```python
from build123d import *

# Parameters (mm, degrees)
SKETCH_1_R          = 3.1
SKETCH_1_R_2        = 1.6
SKETCH_1_W          = 20.4
SKETCH_1_H          = 40.4
EXTRUDE_1_DEPTH     = 4
FILLET_1_R          = 0.2
SKETCH_2_R          = 2.1
CUT_EXTRUDE_1_DEPTH = 4
CUT_EXTRUDE_2_DEPTH = 10
SKETCH_4_W          = 44.796452611
SKETCH_4_H          = 12
CUT_EXTRUDE_3_DEPTH = 10
FILLET_2_R          = 6


with BuildPart() as part:
    # 草图1 → 凸台-拉伸1 (new body)
    with BuildSketch(Plane.XY):
        with BuildLine():
            Line((-13.2, 27), (60.15625, 27))
            ThreePointArc((60.15625, 27), (63.954895943, 25.251198086), (65.096310169, 21.228115599))
            Line((65.096310169, 21.228115599), (62.440060169, 4.228115599))
            ThreePointArc((62.440060169, 4.228115599), (61.816569536, 2.476663431), (60.596300169, 1.074070141))
            Line((60.596300169, 1.074070141), (27.72371786, -24.851859719))
            ThreePointArc((27.72371786, -24.851859719), (24.808418455, -26.447713935), (21.531117522, -27))
            Line((21.531117522, -27), (-13.2, -27))
            ThreePointArc((-13.2, -27), (-20.271067812, -24.071067812), (-23.2, -17))
            Line((-23.2, -17), (-23.2, 17))
            ThreePointArc((-23.2, 17), (-20.271067812, 24.071067812), (-13.2, 27))
        make_face()
        with Locations((33, 2)):
            Circle(SKETCH_1_R, mode=Mode.SUBTRACT)
        with Locations((60, 21)):
            Circle(SKETCH_1_R_2, mode=Mode.SUBTRACT)
        with Locations((57.5, 5)):
            Circle(SKETCH_1_R_2, mode=Mode.SUBTRACT)
        Rectangle(SKETCH_1_W, SKETCH_1_H, mode=Mode.SUBTRACT)
    extrude(amount=EXTRUDE_1_DEPTH)

    # 圆角1
    fillet_1_edges = [part.edges().sort_by_distance(p)[0] for p in [
        (-10.2, 20.2, 2),
        (-10.2, -20.2, 2),
        (10.2, -20.2, 2),
        (10.2, 20.2, 2),
    ]]
    fillet(fillet_1_edges, radius=FILLET_1_R)

    # 草图2 → 切除-拉伸1 (cut)
    with BuildSketch(Plane.XY.offset(4)):
        with Locations((14.95, 11)):
            Circle(SKETCH_2_R)
        with Locations(Location((14.95, -11, 0), (0, 0, 180))):
            Circle(SKETCH_2_R)
        with Locations((-17.95, -11)):
            Circle(SKETCH_2_R)
        with Locations(Location((-17.95, 11, 0), (0, 0, 180))):
            Circle(SKETCH_2_R)
    extrude(amount=-CUT_EXTRUDE_1_DEPTH, mode=Mode.SUBTRACT)

    # 草图3 → 切除-拉伸2 (cut)
    with BuildSketch(Plane.XY.offset(4)):
        with BuildLine():
            Line((25.798016292, 21), (51.43418263, 21))
            ThreePointArc((51.43418263, 21), (53.713370196, 19.950718852), (54.398218731, 17.536869359))
            Line((54.398218731, 17.536869359), (52.852232934, 7.642560256))
            ThreePointArc((52.852232934, 7.642560256), (51.264559821, 5.440053089), (48.549531682, 5.420923567))
            Line((48.549531682, 5.420923567), (24.905572858, 17.210155114))
            ThreePointArc((24.905572858, 17.210155114), (23.851263897, 19.458426781), (25.798016292, 21))
        make_face()
    extrude(amount=-CUT_EXTRUDE_2_DEPTH, mode=Mode.SUBTRACT)

    # 草图4 → 切除-拉伸3 (cut)
    with BuildSketch(Plane.XY.offset(4)):
        with Locations((43.929343828, -21)):
            Rectangle(SKETCH_4_W, SKETCH_4_H)
    extrude(amount=-CUT_EXTRUDE_3_DEPTH, mode=Mode.SUBTRACT)

    # 圆角2
    fillet_2_edges = [part.edges().sort_by_distance(p)[0] for p in [
        (40.215307217, -15, 2),
        (21.531117522, -27, 2),
        (21.531117522, -15, 2),
    ]]
    fillet(fillet_2_edges, radius=FILLET_2_R - 0.0001)  # a hair under: the kernel refuses the full size


solid = part.part
```
Check sheet for the modelled part. Datum: model origin and axes. Units: mm. A direction names the side the tool comes from. Give positions to 0.01 mm unless a question says otherwise; leave off trailing zeros. Write each loop counter-clockwise with the first axis right and the second up, starting at its lowest first coordinate (ties: lowest second). Pieces come first, ordered by that corner, then holes. Notation, with made-up numbers: (78.25, -18) -> (134.25, -18) arc R18 ccw to (134.25, 15) -> close; hole circle Ø11 at (61, -3). An arc over 180 degrees is marked (long way). Use CSV: the item, a comma, the result in double quotes. Start each with the question number.
Q1. Release check for a two-part mould opening along X. For faces 3 (the flat face through (22, 6, 4)), 4 (the cylindrical face through (23.843, 19.422, 2.028)), 5 (the cylindrical face through (63.915, 25.297, 1.972)), 6 (the flat face through (0, -20.2, 2)) record: +X half, -X half, draft (parallel to the pull), parting line (faces both ways), or undercut.
Q2. Scan lines: line 1 along Y through (x, z) = (14.95, 3); line 2 along Y through (x, z) = (-10, 2.45); line 3 along Y through (x, z) = (-17.95, 1.85). Record each from-to range of solid material in increasing order.
Q3. Cross-section at B-B on x = 57.5. Enter the section's corners in (y, z), and give its area (3 significant figures).
Q4. Tool access check on faces 1 (the flat face through (-23.2, 0, 2)), 2 (the cylindrical face through (53.69, 19.98, 2.03)). Record the directions out of +Z, -Z, +X, -X, +Y, -Y that give a thin tool (end or side, any length) a straight path to the whole face; none if there is none.
Q5. Cross-section at D-D on x = -17.95. Enter the section's corners in (y, z), and give its area (3 significant figures).
Q6. Depth check by flat-ended pin: P1, Ø2, axis at y = -6, z = 2.5, coming from the +X side; P2, Ø3.5, axis at x = 33, y = 2, coming from the -Z side; P3, Ø1, axis at y = -20.5, z = 0.5, coming from the -X side; P4, Ø2, axis at y = 11.5, z = 1, coming from the +X side. Enter the tip coordinate at first touch or a pass-through.
Q7. Cross-section at C-C on y = 11. Enter the section's corners in (x, z), and give its area (3 significant figures).
Q8. Cross-section at A-A on y = -11. Enter the section's corners in (x, z), and give its area (3 significant figures).
Working result:
1,face 3,"draft"
1,face 4,"undercut"
1,face 5,"+X half"
1,face 6,"undercut"
2,line 1,"y = -27 to -13.1, -8.9 to 8.9, 13.1 to 27"
2,line 2,"y = -27 to -20.2, 20.2 to 27"
2,line 3,"y = -25.8 to -13.1, -8.9 to 8.9, 13.1 to 25.8"
3,outline,"(-1.37, 0) -> (3.4, 0) -> (3.4, 4) -> (-1.37, 4) -> close; (6.6, 0) -> (27, 0) -> (27, 4) -> (6.6, 4) -> close"
3,area,"101 mm^2"
4,face 1,"+Z, -Z, -X, +Y, -Y"
4,face 2,"+Z, -Z"
5,outline,"(-25.8, 0) -> (-13.1, 0) -> (-13.1, 4) -> (-25.8, 4) -> close; (-8.9, 0) -> (8.9, 0) -> (8.9, 4) -> (-8.9, 4) -> close; (13.1, 0) -> (25.8, 0) -> (25.8, 4) -> (13.1, 4) -> close"
5,area,"173 mm^2"
6,P1,"stops at x = 52.89"
6,P2,"passes through"
6,P3,"stops at x = -22.74"
6,P4,"stops at x = 63.73"
7,outline,"(-23.2, 0) -> (-20.05, 0) -> (-20.05, 4) -> (-23.2, 4) -> close; (-15.85, 0) -> (-10.2, 0) -> (-10.2, 4) -> (-15.85, 4) -> close; (10.2, 0) -> (12.85, 0) -> (12.85, 4) -> (10.2, 4) -> close; (17.05, 0) -> (37.36, 0) -> (37.36, 4) -> (17.05, 4) -> close; (53.38, 0) -> (63.5, 0) -> (63.5, 4) -> (53.38, 4) -> close"
7,area,"168 mm^2"
8,outline,"(-23.2, 0) -> (-20.05, 0) -> (-20.05, 4) -> (-23.2, 4) -> close; (-15.85, 0) -> (-10.2, 0) -> (-10.2, 4) -> (-15.85, 4) -> close; (10.2, 0) -> (12.85, 0) -> (12.85, 4) -> (10.2, 4) -> close; (17.05, 0) -> (45.29, 0) -> (45.29, 4) -> (17.05, 4) -> close"
8,area,"159 mm^2"
